from build123d import *

# Parameters (mm, degrees)
BOSS_EXTRUDE1_DEPTH = 20
SKETCH2_R           = 2
CUT_EXTRUDE1_DEPTH  = 20


with BuildPart() as part:
    # Sketch1 → Boss-Extrude1 (new body)
    with BuildSketch(Plane(origin=(0, 0, 0), x_dir=(1, 0, 0), z_dir=(0, 1, 0))):
        with BuildLine():
            Line((-340, 0), (-900, 0))
            Line((-900, 0), (-779.422863406, 450))
            Line((-779.422863406, 450), (-294.448637287, 170))
            ThreePointArc((-294.448637287, 170), (-328.414780938, 87.998475335), (-340, 0))
        make_face()
    extrude(amount=BOSS_EXTRUDE1_DEPTH)

    # Sketch2 → Cut-Extrude1 (cut)
    with BuildSketch(Plane.XZ):
        with Locations(Location((-850, -5, 0), (0, 0, 270))):
            Circle(SKETCH2_R)
        with Locations(Location((-835, -5, 0), (0, 0, 270))):
            Circle(SKETCH2_R)
        with Locations(Location((-539.91, -5, 0), (0, 0, 270))):
            Circle(SKETCH2_R)
        with Locations(Location((-524.91, -5, 0), (0, 0, 270))):
            Circle(SKETCH2_R)
        with Locations(Location((-399.25, -5, 0), (0, 0, 270))):
            Circle(SKETCH2_R)
        with Locations(Location((-384.25, -5, 0), (0, 0, 270))):
            Circle(SKETCH2_R)
        with Locations(Location((-348.260642461, -195.294872981, 0), (0, 0, 90))):
            Circle(SKETCH2_R)
        with Locations(Location((-335.270261404, -187.794872981, 0), (0, 0, 90))):
            Circle(SKETCH2_R)
        with Locations(Location((-457.0853947, -258.124872981, 0), (0, 0, 90))):
            Circle(SKETCH2_R)
        with Locations(Location((-470.075775757, -265.624872981, 0), (0, 0, 90))):
            Circle(SKETCH2_R)
        with Locations(Location((-725.63121216, -413.169872981, 0), (0, 0, 90))):
            Circle(SKETCH2_R)
        with Locations(Location((-738.621593217, -420.669872981, 0), (0, 0, 90))):
            Circle(SKETCH2_R)
    extrude(amount=-CUT_EXTRUDE1_DEPTH, mode=Mode.SUBTRACT)


solid = part.part
Geometry check sheet. Reference: the model listing, model coordinates, mm. Round coordinates to 2 decimals unless told otherwise and drop trailing zeros. Write each loop counter-clockwise with the first axis right and the second up, starting at its lowest first coordinate (ties: lowest second). Pieces come first, ordered by that corner, then holes. Notation, with made-up numbers: (16, 25.5) -> (28, 25.5) arc R37 ccw to (28, 64.5) -> close; hole circle Ø11 at (-29.75, -29.5). An arc over 180 degrees is marked (long way). One line per item, written item: value. Start each with the question number.
(1) Go/stop test with flat-tipped pins: pin 1 Ø12 at (x, y) = (-403, 13) entering from -Z; pin 2 Ø4 at (y, z) = (3.5, -257.5) entering from -X; pin 3 Ø3 at (x, z) = (-384.25, -5) entering from +Y; pin 4 Ø6.5 at (x, z) = (-738.62, -420.67) entering from +Y. Record where each tip stops, or that it passes through.
(2) Cross-section at B-B, the plane z = -222. Record the cut outline in (x, y).
(3) Cross-section at C-C, the plane x = -807. Record the cut outline in (y, z).
(4) Cross-section at A-A, the plane y = 8. Give the number of separate pieces and of enclosed holes in the cut face, and give its area (3 significant figures).
(5) Scan lines: line 1 (Z direction, x = -524.91, y = 15); line 2 (Z direction, x = -625, y = 8.75); line 3 (X direction, y = 1.25, z = -142). Record each from-to range of solid material in increasing order. Write a range as [from, to].
Answer:
1. pin 1: z = -236.14
1. pin 2: x = -831.54
1. pin 3: through
1. pin 4: y = 20
2. outline: (-840.52, 0) -> (-384.52, 0) -> (-384.52, 20) -> (-840.52, 20) -> close
3. outline: (0, -347.08) -> (20, -347.08) -> (20, 0) -> (0, 0) -> close
4. separate pieces: 1
4. enclosed holes: 12
4. area: 172,000 mm²
5. line 1: [-303.06, -7], [-3, 0]
5. line 2: [-360.84, 0]
5. line 3: [-861.95, -308.93]
